Verification items for the finished model (mm, model axes). Face numbers are marked on the shaded views. A direction names the side the tool comes from. Round coordinates to 2 decimals unless told otherwise and drop trailing zeros. Order: outer loops, then holes, each group sorted by start corner. A loop starts at its lowest first (then second) coordinate and runs counter-clockwise, first axis right, second up. Notation, with made-up numbers: (52.5, 37) -> (108.5, 37) arc R15 ccw to (108.5, 47) -> close; hole circle Ø7 at (63, 24). An arc over 180 degrees is marked (long way). Write item = value, one per line. Start each with the question number.
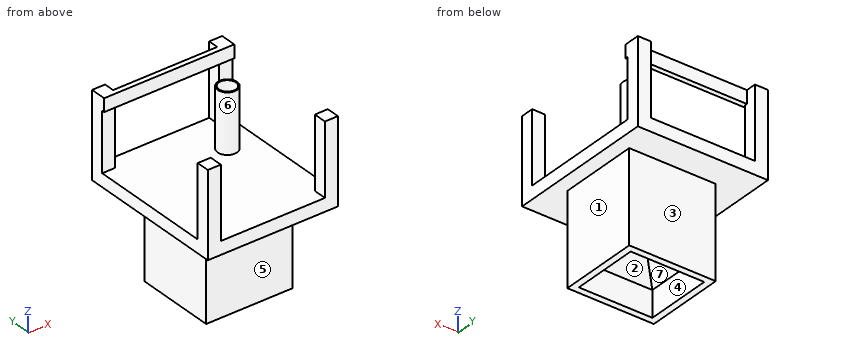
from build123d import *

# Parameters (mm, degrees)
ESQUISSE1_W             = 100
ESQUISSE1_H             = 115
BOSS_EXTRU_2_DEPTH      = 10
ESQUISSE2_W             = 10
ESQUISSE2_H             = 10
BOSS_EXTRU_8_DEPTH      = 55
ESQUISSE9_W             = 10
ESQUISSE9_H             = 10
BOSS_EXTRU_9_DEPTH      = 55
ESQUISSE10_W            = 10
ESQUISSE10_H            = 10
BOSS_EXTRU_10_DEPTH     = 55
ESQUISSE11_W            = 10
ESQUISSE11_H            = 10
BOSS_EXTRU_11_DEPTH     = 55
ESQUISSE14_W            = 100
ESQUISSE14_H            = 10
BOSS_EXTRU_12_DEPTH     = 2
ESQUISSE15_W            = 80
ESQUISSE15_H            = 10
BOSS_EXTRU_13_DEPTH     = 2
ESQUISSE16_R            = 7.5
BOSS_EXTRU_16_DEPTH     = 45
ESQUISSE17_R            = 6.5
ENL_V_MAT_EXTRU_1_DEPTH = 59
ESQUISSE18_W            = 5
ESQUISSE18_H            = 56.5
BOSS_EXTRU_17_DEPTH     = 70
ESQUISSE19_W            = 56.5
ESQUISSE19_H            = 5
BOSS_EXTRU_18_DEPTH     = 70
ESQUISSE21_W            = 5
ESQUISSE21_H            = 56.5
BOSS_EXTRU_19_DEPTH     = 70
ESQUISSE22_W            = 66.5
ESQUISSE22_H            = 5
BOSS_EXTRU_20_DEPTH     = 70
BOSS_EXTRU_21_DEPTH     = 70
ENL_V_MAT_EXTRU_2_DEPTH = 70
BOSS_EXTRU_26_REACH     = 89.238
BOSS_EXTRU_28_REACH     = 86


with BuildPart() as part:
    # Esquisse1 → Boss.-Extru.2 (new body)
    with BuildSketch(Plane.XY):
        with Locations((50, 57.5)):
            Rectangle(ESQUISSE1_W, ESQUISSE1_H)
    extrude(amount=BOSS_EXTRU_2_DEPTH)

    # Esquisse2 → Boss.-Extru.8 (add)
    with BuildSketch(Plane.XY.offset(10)):
        with Locations((5, 110)):
            Rectangle(ESQUISSE2_W, ESQUISSE2_H)
    extrude(amount=BOSS_EXTRU_8_DEPTH)

    # Esquisse9 → Boss.-Extru.9 (add)
    with BuildSketch(Plane.XY.offset(10)):
        with Locations((95, 110)):
            Rectangle(ESQUISSE9_W, ESQUISSE9_H)
    extrude(amount=BOSS_EXTRU_9_DEPTH)

    # Esquisse10 → Boss.-Extru.10 (add)
    with BuildSketch(Plane.XY.offset(10)):
        with Locations((5, 5)):
            Rectangle(ESQUISSE10_W, ESQUISSE10_H)
    extrude(amount=BOSS_EXTRU_10_DEPTH)

    # Esquisse11 → Boss.-Extru.11 (add)
    with BuildSketch(Plane.XY.offset(10)):
        with Locations((95, 5)):
            Rectangle(ESQUISSE11_W, ESQUISSE11_H)
    extrude(amount=BOSS_EXTRU_11_DEPTH)

    # Esquisse14 → Boss.-Extru.12 (add)
    with BuildSketch(Plane.XZ.offset(-105)):
        with Locations((50, 60)):
            Rectangle(ESQUISSE14_W, ESQUISSE14_H)
    extrude(amount=BOSS_EXTRU_12_DEPTH)

    # Esquisse15 → Boss.-Extru.13 (add)
    with BuildSketch(Plane(origin=(0, 105, 0), x_dir=(1, 0, 0), z_dir=(0, 1, 0))):
        with Locations((50, -60)):
            Rectangle(ESQUISSE15_W, ESQUISSE15_H)
    extrude(amount=BOSS_EXTRU_13_DEPTH)

    # Esquisse16 → Boss.-Extru.16 (add)
    with BuildSketch(Plane.XY.offset(10)):
        with Locations((77.5, 80.738453234)):
            Circle(ESQUISSE16_R)
    extrude(amount=BOSS_EXTRU_16_DEPTH)

    # Esquisse17 → Enlèv. mat.-Extru.1 (cut)
    with BuildSketch(Plane.XY.offset(55)):
        with Locations((77.5, 80.738453234)):
            Circle(ESQUISSE17_R)
    extrude(amount=-ENL_V_MAT_EXTRU_1_DEPTH, mode=Mode.SUBTRACT)

    # Esquisse18 → Boss.-Extru.17 (add)
    with BuildSketch(Plane(origin=(0, 0, 0), x_dir=(-1, 0, 0), z_dir=(0, 0, -1))):
        with Locations((-25, 58.988453234)):
            Rectangle(ESQUISSE18_W, ESQUISSE18_H)
    extrude(amount=BOSS_EXTRU_17_DEPTH)

    # Esquisse19 → Boss.-Extru.18 (add)
    with BuildSketch(Plane(origin=(0, 0, 0), x_dir=(-1, 0, 0), z_dir=(0, 0, -1))):
        with Locations((-55.75, 33.238453234)):
            Rectangle(ESQUISSE19_W, ESQUISSE19_H)
    extrude(amount=BOSS_EXTRU_18_DEPTH)

    # Esquisse21 → Boss.-Extru.19 (add)
    with BuildSketch(Plane(origin=(0, 0, 0), x_dir=(-1, 0, 0), z_dir=(0, 0, -1))):
        with Locations((-86.5, 58.988453234)):
            Rectangle(ESQUISSE21_W, ESQUISSE21_H)
    extrude(amount=BOSS_EXTRU_19_DEPTH)

    # Esquisse22 → Boss.-Extru.20 (add)
    with BuildSketch(Plane(origin=(0, 0, 0), x_dir=(-1, 0, 0), z_dir=(0, 0, -1))):
        with Locations((-55.75, 89.738453234)):
            Rectangle(ESQUISSE22_W, ESQUISSE22_H)
    extrude(amount=BOSS_EXTRU_20_DEPTH)

    # Esquisse26 → Boss.-Extru.21 (add)
    with BuildSketch(Plane(origin=(0, 0, -70), x_dir=(-1, 0, 0), z_dir=(0, 0, -1))):
        Polygon((-27.5, 87.238453234), (-84, 35.738453234), (-27.5, 35.738453234), align=None)
    extrude(amount=-BOSS_EXTRU_21_DEPTH)

    # Esquisse23 → Enlèv. mat.-Extru.2 (cut)
    with BuildSketch(Plane(origin=(0, 0, -70), x_dir=(-1, 0, 0), z_dir=(0, 0, -1))):
        Polygon((-27.5, 87.238453234), (-84, 35.738453234), (-27.5, 35.738453234), align=None)
    extrude(amount=-ENL_V_MAT_EXTRU_2_DEPTH, mode=Mode.SUBTRACT)

    # Esquisse24 → Boss.-Extru.26 (add, up to next)
    with BuildSketch(Plane.XZ.offset(-87.238453234), mode=Mode.PRIVATE) as boss_extru_26_sk1:
        Polygon((27.5, -50), (71.5, 0), (27.5, 0), align=None)
    boss_extru_26_tool1 = extrude(boss_extru_26_sk1.sketch, amount=BOSS_EXTRU_26_REACH, mode=Mode.PRIVATE) - part.part
    add(boss_extru_26_tool1.solids().sort_by_distance((42.166667, 87.238453, -16.666667))[0])

    # Esquisse29 → Boss.-Extru.28 (add, up to next)
    with BuildSketch(Plane.ZY.offset(-84), mode=Mode.PRIVATE) as boss_extru_28_sk1:
        Polygon((0, 35.738453234), (-50, 35.738453234), (0, 74.738453234), align=None)
    boss_extru_28_tool1 = extrude(boss_extru_28_sk1.sketch, amount=BOSS_EXTRU_28_REACH, mode=Mode.PRIVATE) - part.part
    add(boss_extru_28_tool1.solids().sort_by_distance((84, 48.738453, -16.666667))[0])


solid = part.part
(1) Depth check by flat-ended pin: pin 1 (4.5 mm diameter, centred on x = 76, y = 86, fed in from -Z); pin 2 (8 mm diameter, centred on y = 19.5, z = -4.5, fed in from -X); pin 3 (1.2 mm diameter, centred on x = 57, y = 105.5, fed in from -Z); pin 4 (5 mm diameter, centred on x = 62, z = -54, fed in from +Y). Enter the tip coordinate at first touch or a pass-through.
(2) Cross-section at A-A (z = 17.5). Enter the section's corners in (x, y).
(3) Set-up check for the marked faces 1, 2 and 3: record each of +Z, -Z, +X, -X, +Y, -Y from which the full face is reachable in a straight line by a thin tool's end or side.
(4) Cross-section at C-C (z = -59.5). Enter the section's corners in (x, y), and give its area (3 significant figures).
(5) Scan lines: line 1 along Y through (x, z) = (77.5, 36.5); line 2 along X through (y, z) = (72, -60); line 3 along Z through (x, y) = (38, 104). Record each from-to range of solid material in increasing order. Write a range as from..to.
(6) Cross-section at D-D (y = 58.5). Enter the section's corners in (x, z).
(7) Cross-section at B-B (x = 60). Enter the section's corners in (y, z), and give its area (3 significant figures).
(8) Draft check along X on the marked faces 4, 5, 6 and 7. Enter one of: +X half, -X half, draft (parallel to the pull), parting line (faces both ways), or undercut.
Outcome:
q1.pin_1 = -70
q1.pin_2 = through
q1.pin_3 = 0
q1.pin_4 = 92.24
q2.outline = (0, 0) -> (10, 0) -> (10, 10) -> (0, 10) -> close; (0, 105) -> (10, 105) -> (10, 115) -> (0, 115) -> close; circle Ø15 at (77.5, 80.74); (90, 0) -> (100, 0) -> (100, 10) -> (90, 10) -> close; (90, 105) -> (100, 105) -> (100, 115) -> (90, 115) -> close; hole circle Ø13 at (77.5, 80.74)
q3.face_1 = -Z, +X, +Y, -Y
q3.face_2 = -Z
q3.face_3 = -Z, +X, -X, +Y
q4.outline = (22.5, 30.74) -> (89, 30.74) -> (89, 92.24) -> (22.5, 92.24) -> close; hole (27.5, 35.74) -> (84, 35.74) -> (84, 87.24) -> (27.5, 87.24) -> close
q4.area = 1,180 mm^2
q5.line_1 = 73.24..74.24, 87.24..88.24
q5.line_2 = 22.5..27.5, 84..89
q5.line_3 = 0..10, 55..65
q6.outline = (0, 0) -> (22.5, 0) -> (22.5, -70) -> (27.5, -70) -> (27.5, -50) -> (53.18, -20.82) -> (84, -20.82) -> (84, -70) -> (89, -70) -> (89, 0) -> (100, 0) -> (100, 10) -> (0, 10) -> close
q7.outline = (0, 0) -> (30.74, 0) -> (30.74, -70) -> (35.74, -70) -> (35.74, -50) -> (64.55, -13.07) -> (87.24, -13.07) -> (87.24, -70) -> (92.24, -70) -> (92.24, 0) -> (115, 0) -> (115, 10) -> (0, 10) -> close; (103, 55) -> (107, 55) -> (107, 65) -> (103, 65) -> close
q7.area = 3,090 mm^2
q8.face_4 = undercut
q8.face_5 = draft
q8.face_6 = parting line
q8.face_7 = undercut
